Can you work these out from the model? Positions are in its coordinate system, mm. Face numbers are marked on the shaded views. Give positions to 0.01 mm unless a question says otherwise; leave off trailing zeros. Order: outer loops, then holes, each group sorted by start corner. A loop starts at its lowest first (then second) coordinate and runs counter-clockwise, first axis right, second up. Notation, with made-up numbers: M 77.5,-36.75 L 89.5,-36.75 A15 ccw 89.5,-13.75 Z; hole C 11.25,4 d3. An arc over 180 degrees is marked long. Use a Markdown table: item, result. Add a question column.
from build123d import *

# Parameters (mm, degrees)
F0_W     = 30.48
F0_H     = 33.02
F1_DEPTH = 4.826
F2_R     = 2.042368
F3_DEPTH = 9.33468
F5_DEPTH = 25


with BuildPart() as f1:
    # F0 (on Top) → F1 (new body)
    with BuildSketch(Plane.XY):
        Rectangle(F0_W, F0_H)
    extrude(amount=-F1_DEPTH)

    # F2 (on face) → F3 (cut)
    with BuildSketch(Plane.XY):
        with Locations((-12.981394, 14.244457)):
            Circle(F2_R)
        with Locations((12.917756, 14.244457)):
            Circle(F2_R)
        with Locations((-12.981394, -14.352153)):
            Circle(F2_R)
        with Locations((12.917756, -14.352153)):
            Circle(F2_R)
    extrude(amount=-F3_DEPTH, mode=Mode.SUBTRACT)

    # F4 (on face) → F5 (cut)
    with BuildSketch(Plane.XY):
        with BuildLine():
            Line((-10.418985, 10.360999), (-14.586995, 10.360999))
            ThreePointArc((-14.586995, 10.360999), (-15.010861, 9.937134), (-14.586995, 9.513268))
            Line((-14.586995, 9.513268), (-10.418985, 9.513268))
            ThreePointArc((-10.418985, 9.513268), (-9.99512, 9.937134), (-10.418985, 10.360999))
        make_face()
        with BuildLine():
            Line((-10.404113, 8.703026), (-14.572124, 8.703026))
            ThreePointArc((-14.572124, 8.703026), (-14.995989, 8.27916), (-14.572124, 7.855295))
            Line((-14.572124, 7.855295), (-10.404113, 7.855295))
            ThreePointArc((-10.404113, 7.855295), (-9.980248, 8.27916), (-10.404113, 8.703026))
        make_face()
        with BuildLine():
            Line((-10.389242, 7.045052), (-14.557252, 7.045052))
            ThreePointArc((-14.557252, 7.045052), (-14.981118, 6.621187), (-14.557252, 6.197322))
            Line((-14.557252, 6.197322), (-10.389242, 6.197322))
            ThreePointArc((-10.389242, 6.197322), (-9.965376, 6.621187), (-10.389242, 7.045052))
        make_face()
        with BuildLine():
            Line((-10.37437, 5.387079), (-14.542381, 5.387079))
            ThreePointArc((-14.542381, 5.387079), (-14.966246, 4.963214), (-14.542381, 4.539348))
            Line((-14.542381, 4.539348), (-10.37437, 4.539348))
            ThreePointArc((-10.37437, 4.539348), (-9.950505, 4.963214), (-10.37437, 5.387079))
        make_face()
        with BuildLine():
            Line((-10.359499, 3.729106), (-14.527509, 3.729106))
            ThreePointArc((-14.527509, 3.729106), (-14.951374, 3.30524), (-14.527509, 2.881375))
            Line((-14.527509, 2.881375), (-10.359499, 2.881375))
            ThreePointArc((-10.359499, 2.881375), (-9.935633, 3.30524), (-10.359499, 3.729106))
        make_face()
        with BuildLine():
            Line((-10.344627, 2.071133), (-14.512637, 2.071133))
            ThreePointArc((-14.512637, 2.071133), (-14.936503, 1.647267), (-14.512637, 1.223402))
            Line((-14.512637, 1.223402), (-10.344627, 1.223402))
            ThreePointArc((-10.344627, 1.223402), (-9.920762, 1.647267), (-10.344627, 2.071133))
        make_face()
        with BuildLine():
            Line((-10.329755, 0.413159), (-14.497766, 0.413159))
            ThreePointArc((-14.497766, 0.413159), (-14.921631, -0.010706), (-14.497766, -0.434572))
            Line((-14.497766, -0.434572), (-10.329755, -0.434572))
            ThreePointArc((-10.329755, -0.434572), (-9.90589, -0.010706), (-10.329755, 0.413159))
        make_face()
        with BuildLine():
            Line((-10.314884, -1.244814), (-14.482894, -1.244814))
            ThreePointArc((-14.482894, -1.244814), (-14.90676, -1.668679), (-14.482894, -2.092545))
            Line((-14.482894, -2.092545), (-10.314884, -2.092545))
            ThreePointArc((-10.314884, -2.092545), (-9.891018, -1.668679), (-10.314884, -1.244814))
        make_face()
        with BuildLine():
            Line((-10.300012, -2.902787), (-14.468023, -2.902787))
            ThreePointArc((-14.468023, -2.902787), (-14.891888, -3.326653), (-14.468023, -3.750518))
            Line((-14.468023, -3.750518), (-10.300012, -3.750518))
            ThreePointArc((-10.300012, -3.750518), (-9.876147, -3.326653), (-10.300012, -2.902787))
        make_face()
        with BuildLine():
            Line((-10.285141, -4.560761), (-14.453151, -4.560761))
            ThreePointArc((-14.453151, -4.560761), (-14.877016, -4.984626), (-14.453151, -5.408491))
            Line((-14.453151, -5.408491), (-10.285141, -5.408491))
            ThreePointArc((-10.285141, -5.408491), (-9.861275, -4.984626), (-10.285141, -4.560761))
        make_face()
        with BuildLine():
            ThreePointArc((14.586995, 9.513268), (15.010861, 9.937134), (14.586995, 10.360999))
            Line((14.586995, 10.360999), (10.418985, 10.360999))
            ThreePointArc((10.418985, 10.360999), (9.99512, 9.937134), (10.418985, 9.513268))
            Line((10.418985, 9.513268), (14.586995, 9.513268))
        make_face()
        with BuildLine():
            ThreePointArc((14.572124, 7.855295), (14.995989, 8.27916), (14.572124, 8.703026))
            Line((14.572124, 8.703026), (10.404113, 8.703026))
            ThreePointArc((10.404113, 8.703026), (9.980248, 8.27916), (10.404113, 7.855295))
            Line((10.404113, 7.855295), (14.572124, 7.855295))
        make_face()
        with BuildLine():
            ThreePointArc((14.557252, 6.197322), (14.981118, 6.621187), (14.557252, 7.045052))
            Line((14.557252, 7.045052), (10.389242, 7.045052))
            ThreePointArc((10.389242, 7.045052), (9.965376, 6.621187), (10.389242, 6.197322))
            Line((10.389242, 6.197322), (14.557252, 6.197322))
        make_face()
        with BuildLine():
            ThreePointArc((14.542381, 4.539348), (14.966246, 4.963214), (14.542381, 5.387079))
            Line((14.542381, 5.387079), (10.37437, 5.387079))
            ThreePointArc((10.37437, 5.387079), (9.950505, 4.963214), (10.37437, 4.539348))
            Line((10.37437, 4.539348), (14.542381, 4.539348))
        make_face()
        with BuildLine():
            ThreePointArc((14.527509, 2.881375), (14.951374, 3.30524), (14.527509, 3.729106))
            Line((14.527509, 3.729106), (10.359499, 3.729106))
            ThreePointArc((10.359499, 3.729106), (9.935633, 3.30524), (10.359499, 2.881375))
            Line((10.359499, 2.881375), (14.527509, 2.881375))
        make_face()
        with BuildLine():
            ThreePointArc((14.512637, 1.223402), (14.936503, 1.647267), (14.512637, 2.071133))
            Line((14.512637, 2.071133), (10.344627, 2.071133))
            ThreePointArc((10.344627, 2.071133), (9.920762, 1.647267), (10.344627, 1.223402))
            Line((10.344627, 1.223402), (14.512637, 1.223402))
        make_face()
        with BuildLine():
            ThreePointArc((14.497766, -0.434572), (14.921631, -0.010706), (14.497766, 0.413159))
            Line((14.497766, 0.413159), (10.329755, 0.413159))
            ThreePointArc((10.329755, 0.413159), (9.90589, -0.010706), (10.329755, -0.434572))
            Line((10.329755, -0.434572), (14.497766, -0.434572))
        make_face()
        with BuildLine():
            ThreePointArc((14.482894, -2.092545), (14.90676, -1.668679), (14.482894, -1.244814))
            Line((14.482894, -1.244814), (10.314884, -1.244814))
            ThreePointArc((10.314884, -1.244814), (9.891018, -1.668679), (10.314884, -2.092545))
            Line((10.314884, -2.092545), (14.482894, -2.092545))
        make_face()
        with BuildLine():
            ThreePointArc((14.468023, -3.750518), (14.891888, -3.326653), (14.468023, -2.902787))
            Line((14.468023, -2.902787), (10.300012, -2.902787))
            ThreePointArc((10.300012, -2.902787), (9.876147, -3.326653), (10.300012, -3.750518))
            Line((10.300012, -3.750518), (14.468023, -3.750518))
        make_face()
        with BuildLine():
            ThreePointArc((14.453151, -5.408491), (14.877016, -4.984626), (14.453151, -4.560761))
            Line((14.453151, -4.560761), (10.285141, -4.560761))
            ThreePointArc((10.285141, -4.560761), (9.861275, -4.984626), (10.285141, -5.408491))
            Line((10.285141, -5.408491), (14.453151, -5.408491))
        make_face()
    extrude(amount=-F5_DEPTH, mode=Mode.SUBTRACT)


solid = f1.part
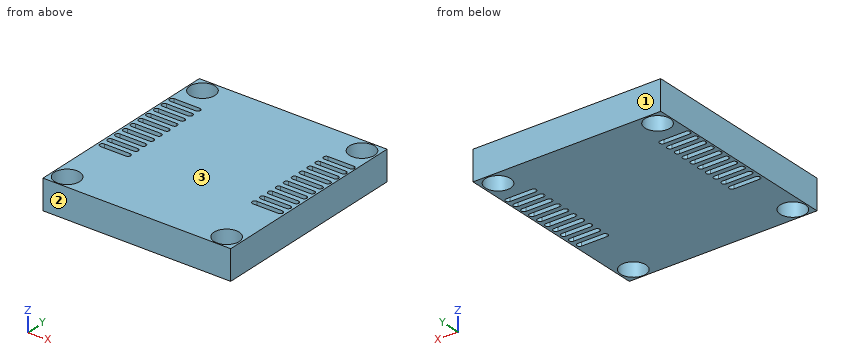
1. If we section it at A-A, the plane y = 13.5: List the corners of the cut face in (x, z) for me.
2. We'd pull the mould along Y, two halves only. Please class the marked faces 1, 2 and 3: +Y half, -Y half, draft (parallel to the pull), parting line (faces both ways), or undercut.
3. Will this pin go through, and if not, where does the flat tip stop? pin 1 (4 mm diameter, centred on x = 2, y = 4, fed in from +Z).
4. I need wall thicknesses on L1, parallel to X at y = 1.5, z = -2.65; L2, parallel to X at y = 13, z = -3.65. Which ranges of each line are inside material? Lowest first, please. Write a range as [from, to].
5. If we section it at B-B, the plane z = -0.75: State how many separate pieces and enclosed holes the cut face has, then the cut area to 3 significant figures.
Geometry results:
| question | item | result |
|---|---|---|
| 1 | outline | M -15.24,-4.83 L -14.88,-4.83 L -14.88,0 L -15.24,0 Z; M -11.08,-4.83 L 11.02,-4.83 L 11.02,0 L -11.08,0 Z; M 14.82,-4.83 L 15.24,-4.83 L 15.24,0 L 14.82,0 Z |
| 2 | face 1 | +Y half |
| 2 | face 2 | -Y half |
| 2 | face 3 | draft |
| 3 | pin 1 | stops at z = 0 |
| 4 | L1 | x = [-15.24, -14.91], [-9.95, 9.95], [14.91, 15.24] |
| 4 | L2 | x = [-15.24, -14.6], [-11.36, 11.3], [14.54, 15.24] |
| 5 | separate pieces | 1 |
| 5 | enclosed holes | 24 |
| 5 | area | 872 mm^2 |
